```python
from build123d import *

# Parameters (mm, degrees)
SKETCH6_R          = 40
CUT_EXTRUDE3_DEPTH = 59.294788524860515
SKETCH10_R         = 35.361197
CUT_EXTRUDE6_DEPTH = 199.0000000000001
SKETCH13_R         = 11.999999999999975
CUT_EXTRUDE7_DEPTH = 65


with BuildPart() as part:
    # Sketch2 → Revolve2 (revolve)
    with BuildSketch(Plane.XY):
        with BuildLine():
            Line((0, 100), (2.776e-14, -100))
            ThreePointArc((2.776e-14, -100), (-100, 1.225e-14), (0, 100))
        make_face()
    revolve(axis=Axis((0, 100, 0), (1.4e-16, -1, 0)))

    # Sketch6 → Cut-Extrude3 (cut)
    with BuildSketch(Plane(origin=(-2.5379788603345292, 100, 26.23220958860291), x_dir=(-1, 0, 0), z_dir=(0, -1, 0))):
        with Locations(Location((0, 0, 0), (0, 0, 139.019257533))):
            Circle(SKETCH6_R)
    extrude(amount=CUT_EXTRUDE3_DEPTH, mode=Mode.SUBTRACT)

    # Sketch10 → Cut-Extrude6 (cut)
    with BuildSketch(Plane(origin=(-2.879635505276285, 100, -0.1784267377198251), x_dir=(1, 0, 0), z_dir=(0, 1, 0))):
        with Locations((0, 71.71708866685675)):
            Circle(SKETCH10_R)
    extrude(amount=-CUT_EXTRUDE6_DEPTH, mode=Mode.SUBTRACT)

    # Sketch13 → Cut-Extrude7 (cut, symmetric)
    with BuildSketch(Plane(origin=(0, 0, 0), x_dir=(0, 0, -1), z_dir=(1, 0, 0))):
        with Locations((60, 0)):
            Circle(SKETCH13_R)
    extrude(amount=CUT_EXTRUDE7_DEPTH, both=True, mode=Mode.SUBTRACT)


solid = part.part
```
Here's how the part is built. I have some questions about the finished solid (model axes, mm). A direction names the side the tool comes from. Coordinates: 2 decimals unless noted, no trailing zeros. Loops run counter-clockwise (first coordinate to the right, second up) from the corner with the lowest first, then second, coordinate; pieces in that order, holes last. Notation, with made-up numbers: (16.5, 31.5) - (29.5, 31.5) arc R13 cw to (29.5, 42.5) - close; hole circle Ø7 at (14, 28). An arc over 180 degrees is marked (long way). Return JSON: item names as keys, results as strings. Group by question number.
Item 1: If we section it at D-D on z = 26: Write out the boundary of the cut face in (x, y), and give its area (3 significant figures).
Item 2: If we section it at B-B on y = 0: Write out the boundary of the cut face in (x, z), and give its area (3 significant figures).
Item 3: On a 3-axis mill with a long thin cutter (end or side, diameter ignored), from which of +Z, -Z, +X, -X, +Y, -Y can I reach the whole of each face in a straight line? I mean faces 1 (the face through (15.309, 63.811, -9.565)), 2 (the face through (-65, 0, -60)), 3 (the face through (-2.627, 1.303, -36.535)). Say none if no direction works.
Item 4: Will these pins go through, and if not, where does the flat tip stop? P1, Ø7, axis at y = 4.5, z = -56, coming from the -X side; P2, Ø8, axis at x = -46.5, z = 0, coming from the -Y side; P3, Ø8, axis at x = 77, z = -2.5, coming from the -Y side.
Item 5: I need wall thicknesses on line 1 (X direction, y = -52.5, z = -60); line 2 (Z direction, x = -48.5, y = 0); line 3 (Z direction, x = -5.5, y = 58). Which ranges of each line are inside material? Lowest first, please. Write a range as from..to.
Item 6: If we section it at C-C on x = -51.5: Write out the boundary of the cut face in (y, z), and give its area (3 significant figures).
Item 7: If we section it at A-A on z = -60: Write out the boundary of the cut face in (x, y), and give its area (3 significant figures).
Calculated:
{
 "1": {"outline": "(-42.54, 40.71) - (-42.54, 86.69) arc R96.56 ccw (long way) to (37.46, 89) - (37.46, 40.71) - close", "area": "25,100 mm^2"},
 "2": {"outline": "(-65, -72) - (-65, -48) - (-28.95, -48) arc R35.36 cw to (23.19, -48) - (65, -48) - (65, -72) - (32.48, -72) arc R35.36 cw to (21.29, -97.71) arc R100 ccw (long way) to (-29.04, -95.69) arc R35.36 cw to (-38.24, -72) - close", "area": "26,200 mm^2"},
 "3": {"face 1": "+Y", "face 2": "none", "face 3": "+Y, -Y"},
 "4": {"P1": "stops at x = -85", "P2": "stops at y = -90.52", "P3": "stops at y = -68.3"},
 "5": {"line 1": "x = -60.36..-36.18, 30.42..60.36", "line 2": "z = -87.45..-72, -48..87.45", "line 3": "z = -36.63..-13.66, 66.12..81.28"},
 "6": {"outline": "circle Ø171.44 at (0, 0); hole circle Ø24 at (0, -60)", "area": "22,600 mm^2"},
 "7": {"outline": "(-65, -12) - (-65, 12) - (-36.18, 12) - (-36.18, 71.35) arc R80 ccw to (-36.18, -71.35) - (-36.18, -12) - close; (30.42, -73.99) arc R80 ccw to (30.42, 73.99) - (30.42, 12) - (65, 12) - (65, -12) - (30.42, -12) - close", "area": "8,250 mm^2"}
}
